Job drawing, mm, ordinate dimensions from the low corner. One solid piece. A direction names the side the tool comes from. Round coordinates to 2 decimals unless told otherwise and drop trailing zeros. Loops run counter-clockwise (first coordinate to the right, second up) from the corner with the lowest first, then second, coordinate; pieces in that order, holes last. Notation, with made-up numbers: M -9.75,27.5 L 46.25,27.5 A21 cw 46.25,59.5 Z; hole C 3.5,-24 d5. An arc over 180 degrees is marked long. One line per item, written item: value.
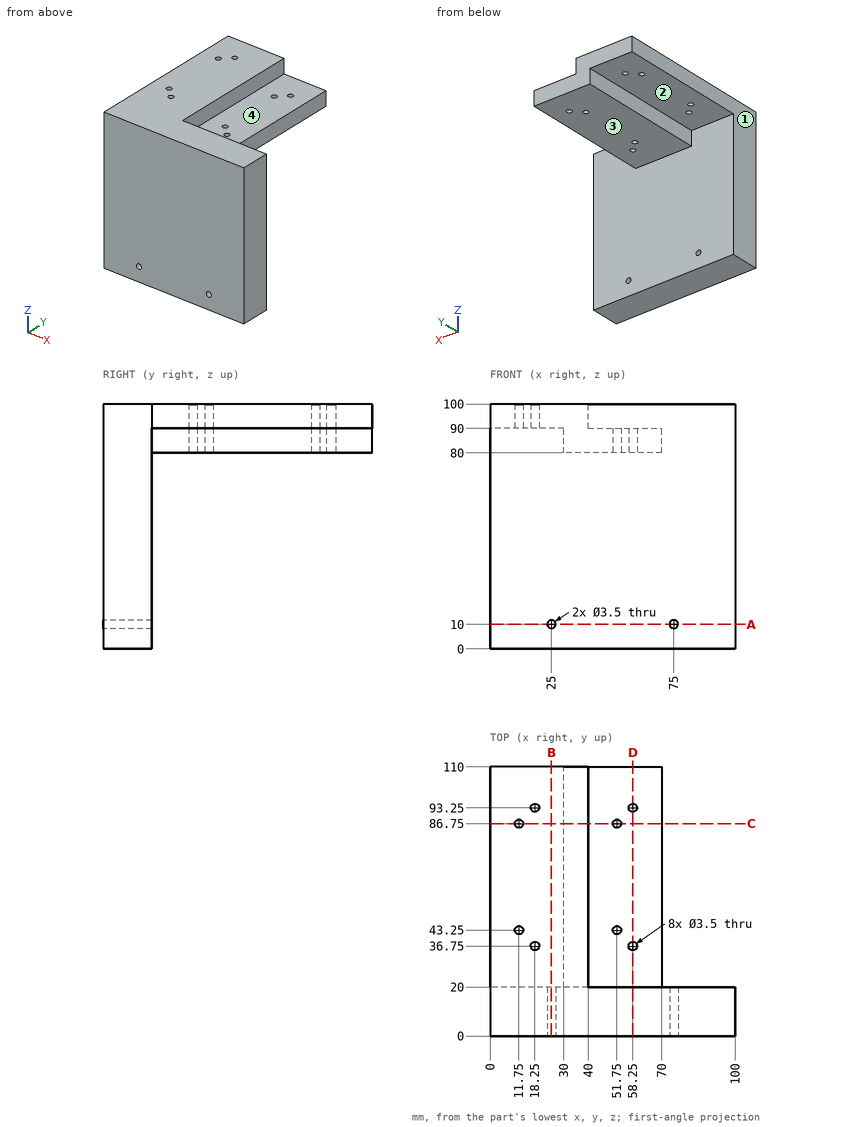
Item 1: Slice it at C-C, the plane y = 86.75. Give the cut face in (x, z).
Check values:
outline: M 0,90 L 10,90 L 10,100 L 0,100 Z; M 13.5,90 L 30,90 L 30,80 L 50,80 L 50,90 L 40,90 L 40,100 L 13.5,100 Z; M 53.5,80 L 70,80 L 70,90 L 53.5,90 Z
Item 2: Wall check: line 1 along Y through (x, z) = (58, 85); line 2 along Y through (x, z) = (51.75, 86.75); line 3 along Z through (x, y) = (25, 13). Give the ranges that are in metal, low to high.
Check values:
line 1: y = 0 to 35.02, 38.48 to 91.52, 94.98 to 110
line 2: y = 0 to 41.5, 45 to 85, 88.5 to 110
line 3: z = 0 to 8.25, 11.75 to 100
Item 3: Slice it at B-B, the plane x = 25. Give the cut face in (y, z).
Check values:
outline: M 0,0 L 20,0 L 20,8.25 L 0,8.25 Z; M 0,11.75 L 20,11.75 L 20,90 L 110,90 L 110,100 L 0,100 Z
Item 4: Slice it at A-A, the plane z = 10. Give the cut face in (x, y), and give its area (3 significant figures).
Check values:
outline: M 0,0 L 23.25,0 L 23.25,20 L 0,20 Z; M 26.75,0 L 73.25,0 L 73.25,20 L 26.75,20 Z; M 76.75,0 L 100,0 L 100,20 L 76.75,20 Z
area: 1,860 mm2
Item 5: Which spindle directions (+Z, -Z, +X, -X, +Y, -Y) get a long thin tool onto all of the face, cutting with end or side? Do the marked faces 1, 2, 3 and 4. Say none if no direction does.
Check values:
face 1: +Z, -Z, -X, +Y, -Y
face 2: -Z, -X, +Y
face 3: -Z, +X, -X, +Y
face 4: +Z, +X, +Y
Item 6: Slice it at D-D, the plane x = 58.25. Give the cut face in (y, z).
Check values:
outline: M 0,0 L 20,0 L 20,80 L 35,80 L 35,90 L 20,90 L 20,100 L 0,100 Z; M 38.5,80 L 91.5,80 L 91.5,90 L 38.5,90 Z; M 95,80 L 110,80 L 110,90 L 95,90 Z
Item 7: Drop flat-ended pins along their axis: P1, Ø5.5, axis at x = 75, z = 10, coming from the -Y side; P2, Ø4.5, axis at x = 51.75, y = 86.75, coming from the -Z side; P3, Ø24, axis at x = 61.5, y = 69, coming from the +Z side; P4, Ø4, axis at x = 11.75, y = 43.25, coming from the -Z side. Give the stop position or say it passes through.
Check values:
P1: stops at y = 0
P2: stops at z = 80
P3: stops at z = 90
P4: stops at z = 90
